from build123d import *

# Parameters (mm, degrees)
SKETCH_1_W          = 36
SKETCH_1_H          = 32
SKETCH_1_R          = 1.5
EXTRUDE_1_DEPTH     = 4
EXTRUDE_2_DEPTH     = 32
SKETCH_8_R          = 1.5
CUT_EXTRUDE_1_DEPTH = 5
SKETCH1_W           = 4
SKETCH1_H           = 32
BOSS_EXTRUDE1_DEPTH = 3
SKETCH2_W           = 5
SKETCH2_H           = 32
BOSS_EXTRUDE2_DEPTH = 12
CUT_EXTRUDE1_DEPTH  = 5
BOSS_EXTRUDE5_DEPTH = 5
SKETCH7_W           = 15
SKETCH7_H           = 32
SKETCH7_R           = 1.5
BOSS_EXTRUDE6_DEPTH = 3
CUT_EXTRUDE2_DEPTH  = 0.25


with BuildPart() as part:
    # Эскиз1 → Бобышка-Вытянуть1 (new body)
    with BuildSketch(Plane.XY):
        with Locations((18, 16)):
            Rectangle(SKETCH_1_W, SKETCH_1_H)
        with Locations((8, 26)):
            Circle(SKETCH_1_R, mode=Mode.SUBTRACT)
        with Locations((28, 26)):
            Circle(SKETCH_1_R, mode=Mode.SUBTRACT)
        with Locations((8, 6)):
            Circle(SKETCH_1_R, mode=Mode.SUBTRACT)
        with Locations((28, 6)):
            Circle(SKETCH_1_R, mode=Mode.SUBTRACT)
    extrude(amount=EXTRUDE_1_DEPTH)

    # Эскиз7 → Бобышка-Вытянуть2 (add)
    with BuildSketch(Plane(origin=(0, 32, 0), x_dir=(1, 0, 0), z_dir=(0, 1, 0))):
        Polygon((0, 0), (-1.2, 0), (-1.2, 15), (-5.2, 15), (-5.2, -19), (-1.2, -19), (-1.2, -4), (0, -4), align=None)
    extrude(amount=-EXTRUDE_2_DEPTH)

    # Эскиз8 → Вырез-Вытянуть1 (cut, through all)
    with BuildSketch(Plane(origin=(-1.2, 0, 0), x_dir=(0, 0, -1), z_dir=(1, 0, 0))):
        with Locations((8, 24)):
            Circle(SKETCH_8_R)
        with Locations((8, 8)):
            Circle(SKETCH_8_R)
        with Locations((-12, 8)):
            Circle(SKETCH_8_R)
        with Locations((-12, 24)):
            Circle(SKETCH_8_R)
    extrude(amount=-CUT_EXTRUDE_1_DEPTH, mode=Mode.SUBTRACT)

    # Sketch1 → Boss-Extrude1 (add)
    with BuildSketch(Plane(origin=(36, 0, 0), x_dir=(0, 0, -1), z_dir=(1, 0, 0))):
        with Locations((-2, 16)):
            Rectangle(SKETCH1_W, SKETCH1_H)
    extrude(amount=BOSS_EXTRUDE1_DEPTH)

    # Sketch2 → Boss-Extrude2 (add)
    with BuildSketch(Plane(origin=(0, 0, 0), x_dir=(-1, 0, 0), z_dir=(0, 0, -1))):
        with Locations((-36.5, 16)):
            Rectangle(SKETCH2_W, SKETCH2_H)
    extrude(amount=BOSS_EXTRUDE2_DEPTH)

    # Sketch3 → Cut-Extrude1 (cut)
    with BuildSketch(Plane(origin=(39, 0, 0), x_dir=(0, 0, -1), z_dir=(1, 0, 0))):
        Polygon((7, 32), (12, 32), (12, 23.339745962), align=None)
        Polygon((12, 8.660254038), (7, 0), (12, 0), align=None)
    extrude(amount=-CUT_EXTRUDE1_DEPTH, mode=Mode.SUBTRACT)

    # Sketch6 → Boss-Extrude5 (add)
    with BuildSketch(Plane(origin=(39, 0, 0), x_dir=(0, 0, -1), z_dir=(1, 0, 0))):
        Polygon((-16, 8.660254038), (-11, 0), (-4, 0), (-4, 32), (-11, 32), (-16, 23.339745962), align=None)
    extrude(amount=-BOSS_EXTRUDE5_DEPTH)

    # Sketch7 → Boss-Extrude6 (add)
    with BuildSketch(Plane(origin=(-1.2, 0, 0), x_dir=(0, 0, -1), z_dir=(1, 0, 0))):
        with Locations((7.5, 16)):
            Rectangle(SKETCH7_W, SKETCH7_H)
        with Locations((8, 24)):
            Circle(SKETCH7_R, mode=Mode.SUBTRACT)
        with Locations((8, 8)):
            Circle(SKETCH7_R, mode=Mode.SUBTRACT)
        with Locations((-11.5, 16)):
            Rectangle(SKETCH7_W, SKETCH7_H)
        with Locations((-12, 24)):
            Circle(SKETCH7_R, mode=Mode.SUBTRACT)
        with Locations((-12, 8)):
            Circle(SKETCH7_R, mode=Mode.SUBTRACT)
    extrude(amount=BOSS_EXTRUDE6_DEPTH)

    # Sketch8 → Cut-Extrude2 (cut)
    with BuildSketch(Plane.ZY.offset(-34)):
        Polygon((-12, 23.339745962), (-12, 8.660254038), (-7, 0), (0, 0), (0, 32), (-7, 32), align=None)
        Polygon((4, 32), (4, 0), (11, 0), (16, 8.660254038), (16, 23.339745962), (11, 32), align=None)
    extrude(amount=-CUT_EXTRUDE2_DEPTH, mode=Mode.SUBTRACT)


solid = part.part
Verification items for the finished model (mm, model axes). A direction names the side the tool comes from. Round coordinates to 2 decimals unless told otherwise and drop trailing zeros. Write each loop counter-clockwise with the first axis right and the second up, starting at its lowest first coordinate (ties: lowest second). Pieces come first, ordered by that corner, then holes.
(1) Section check D-D (y = 18). Enter the section's corners in (x, z).
Returned:
outline: (-5.2, -15) - (1.8, -15) - (1.8, 0) - (34.25, 0) - (34.25, -12) - (39, -12) - (39, 16) - (34.25, 16) - (34.25, 4) - (1.8, 4) - (1.8, 19) - (-5.2, 19) - close
(2) Section check B-B (z = -5.5). Enter the section's corners in (x, y), plus the area to 3 significant figures.
Returned:
outline: (-5.2, 0) - (1.8, 0) - (1.8, 32) - (-5.2, 32) - close; (34.25, 0) - (39, 0) - (39, 32) - (34.25, 32) - close
area: 376 mm2
(3) Material ranges on line 1 (Y direction, x = 28, z = 2.6); line 2 (Y direction, x = -3, z = -8); line 3 (X direction, y = 27.5, z = -7), recorded low to high.
Returned:
line 1: y = 0 to 4.5, 7.5 to 24.5, 27.5 to 32
line 2: y = 0 to 6.5, 9.5 to 22.5, 25.5 to 32
line 3: x = -5.2 to 1.8, 34.25 to 39
(4) Section check C-C (z = 12). Enter the section's corners in (x, y).
Returned:
outline: (-5.2, 0) - (1.8, 0) - (1.8, 6.5) - (-5.2, 6.5) - close; (-5.2, 9.5) - (1.8, 9.5) - (1.8, 22.5) - (-5.2, 22.5) - close; (-5.2, 25.5) - (1.8, 25.5) - (1.8, 32) - (-5.2, 32) - close; (34.25, 1.73) - (39, 1.73) - (39, 30.27) - (34.25, 30.27) - close
(5) Section check A-A (x = 8). Enter the section's corners in (y, z).
Returned:
outline: (0, 0) - (4.5, 0) - (4.5, 4) - (0, 4) - close; (7.5, 0) - (24.5, 0) - (24.5, 4) - (7.5, 4) - close; (27.5, 0) - (32, 0) - (32, 4) - (27.5, 4) - close
(6) Access from +Z, -Z, +X, -X, +Y, -Y to the whole of each face (thin tool, end or side, straight path). Record for faces 5 (the flat face through (37, 16, 16)), 6 (the flat face through (36.658, 4.391, -9.535)), 7 (the flat face through (36.658, 27.609, -9.535)), 8 (the flat face through (34.25, 16, -6)).
Returned:
face 5: +Z, +X, +Y, -Y
face 6: -Z, +X, -Y
face 7: -Z, +X, +Y
face 8: -Z, +Y, -Y
(7) Depth check by flat-ended pin: pin 1 Ø2.5 at (x, y) = (36, 14) entering from +Z; pin 2 Ø1.8 at (x, y) = (28, 6) entering from -Z; pin 3 Ø1.5 at (x, y) = (18, 10.5) entering from -Z; pin 4 Ø3 at (x, y) = (24.5, 26.5) entering from +Z. Enter the tip coordinate at first touch or a pass-through.
Returned:
pin 1: stops at z = 16
pin 2: passes through
pin 3: stops at z = 0
pin 4: stops at z = 4
(8) Mould release check, pull along Y, two halves, no side actions. Record for faces 1 (the cylindrical face through (6.8, 5.1, 2)), 2 (the flat face through (39, 16, 2)), 3 (the flat face through (36.658, 4.391, 13.535)), 4 (the flat face through (36.658, 27.73, 13.465)): pulls with the +Y half, pulls with the -Y half, needs draft (parallel to the pull), parting line crosses it, or undercut.
Returned:
face 1: undercut
face 2: needs draft
face 3: pulls with the -Y half
face 4: pulls with the +Y half
